```python
from build123d import *

# Parameters (mm, degrees)
SKETCH1_R           = 6.35
BOSS_EXTRUDE1_DEPTH = 6.0833
SKETCH4_R           = 7.62
BOSS_EXTRUDE2_DEPTH = 5.08
BOSS_EXTRUDE3_DEPTH = 6.35
SKETCH13_R          = 6.35
BOSS_EXTRUDE4_DEPTH = 72.46112


with BuildPart() as part:
    # Sketch1 → Boss-Extrude1 (new body)
    with BuildSketch(Plane.XY):
        Circle(SKETCH1_R)
    extrude(amount=BOSS_EXTRUDE1_DEPTH)

    # Sketch4 → Boss-Extrude2 (add)
    with BuildSketch(Plane(origin=(0, 0, 0), x_dir=(-1, 0, 0), z_dir=(0, 0, -1))):
        Circle(SKETCH4_R)
    extrude(amount=BOSS_EXTRUDE2_DEPTH)

    # Sketch12 → Boss-Extrude3 (add)
    with BuildSketch(Plane.XY.offset(6.0833)):
        with BuildLine():
            Line((0, -6.35), (6.35, 0))
            ThreePointArc((6.35, 0), (-4.490128061, 4.490128061), (0, -6.35))
        make_face()
    extrude(amount=BOSS_EXTRUDE3_DEPTH)

    # Sketch13 → Boss-Extrude4 (add)
    with BuildSketch(Plane.XY.offset(12.4333)):
        Circle(SKETCH13_R)
    extrude(amount=BOSS_EXTRUDE4_DEPTH)


solid = part.part
```
Verification items for the finished model (mm, model axes). A direction names the side the tool comes from. Coordinates: 2 decimals unless noted, no trailing zeros. Loops run counter-clockwise (first coordinate to the right, second up) from the corner with the lowest first, then second, coordinate; pieces in that order, holes last. Notation, with made-up numbers: (-30.75, 33) - (0.25, 33) arc R21 ccw to (0.25, 52) - close; hole circle Ø1 at (-36.5, 26). An arc over 180 degrees is marked (long way). Answer as a JSON object with one key per item and string values.
(1) Cross-section at A-A, the plane y = -0.75. Record the boundary of the cut face in (x, z), then the cut area to 3 significant figures.
Response:
{"outline": "(-7.58, -5.08) - (7.58, -5.08) - (7.58, 0) - (6.31, 0) - (6.31, 6.08) - (5.6, 6.08) - (5.6, 12.43) - (6.31, 12.43) - (6.31, 84.89) - (-6.31, 84.89) - (-6.31, 0) - (-7.58, 0) - close", "area": "1,140 mm²"}
(2) Mould release check, pull along Z, two halves, no side actions. Record for faces 4 (the cylindrical face through (1.65, -7.44, -2.5)), 5 (the flat face through (4, -4, 12.433)), 6 (the flat face through (0, 0, 84.894)): pulls with the +Z half, pulls with the -Z half, needs draft (parallel to the pull), parting line crosses it, or undercut.
Response:
{"face 4": "needs draft", "face 5": "undercut", "face 6": "pulls with the +Z half"}
(3) Cross-section at C-C, the plane z = 63.5. Record the boundary of the cut face in (x, y), then the cut area to 3 significant figures.
Response:
{"outline": "circle Ø12.7 at (0, 0)", "area": "127 mm²"}
(4) Go/stop test with flat-tipped pins: pin 1 Ø1 at (x, y) = (5.5, -4) entering from +Z; pin 2 Ø4 at (y, z) = (-2.5, 65.5) entering from -X; pin 3 Ø8 at (y, z) = (-3, 25.5) entering from +X; pin 4 Ø2 at (y, z) = (-3, 59) entering from -X. Record where each tip stops, or that it passes through.
Response:
{"pin 1": "stops at z = 84.89", "pin 2": "stops at x = -6.33", "pin 3": "stops at x = 6.35", "pin 4": "stops at x = -6.03"}
(5) Access from +Z, -Z, +X, -X, +Y, -Y to the whole of each face (thin tool, end or side, straight path). Record for faces 1 (the flat face through (0, 0, -5.08)), 2 (the flat face through (4, -4, 6.083)), 3 (the flat face through (3, 6, 0)).
Response:
{"face 1": "-Z, +X, -X, +Y, -Y", "face 2": "+X, -Y", "face 3": "+Z"}
(6) Cross-section at B-B, the plane x = 1.25. Record the boundary of the cut face in (y, z).
Response:
{"outline": "(-7.52, -5.08) - (7.52, -5.08) - (7.52, 0) - (6.23, 0) - (6.23, 84.89) - (-6.23, 84.89) - (-6.23, 12.43) - (-5.1, 12.43) - (-5.1, 6.08) - (-6.23, 6.08) - (-6.23, 0) - (-7.52, 0) - close"}
(7) Cross-section at D-D, the plane y = 3.75. Record the boundary of the cut face in (x, z).
Response:
{"outline": "(-6.63, -5.08) - (6.63, -5.08) - (6.63, 0) - (5.12, 0) - (5.12, 84.89) - (-5.12, 84.89) - (-5.12, 0) - (-6.63, 0) - close"}
(8) Scan lines: line 1 along Z through (x, y) = (-6.25, 3.25); line 2 along Y through (x, z) = (0, 78); line 3 along Y through (x, z) = (-2, 3.5). Record each from-to range of solid material in increasing order.
Response:
{"line 1": "z = -5.08 to 0", "line 2": "y = -6.35 to 6.35", "line 3": "y = -6.03 to 6.03"}
